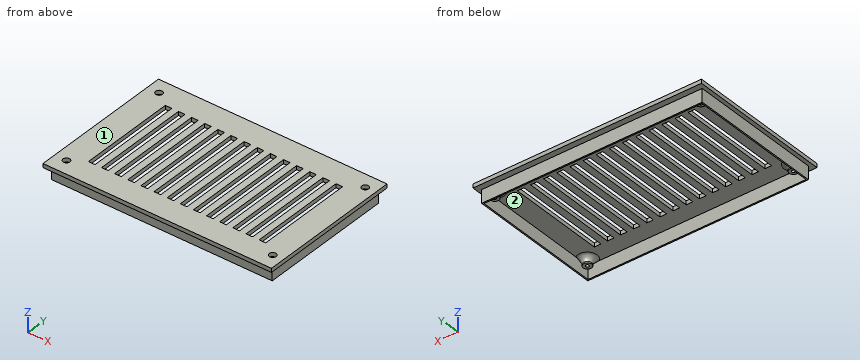
from build123d import *

# Parameters (mm, degrees)
SKETCH1_W           = 174
SKETCH1_H           = 111
SKETCH1_R           = 2.6
SKETCH1_W_2         = 5
SKETCH1_H_2         = 73.910542587
BOSS_EXTRUDE1_DEPTH = 1.5
SKETCH2_R           = 3.25
SKETCH2_R_2         = 1.25
BOSS_EXTRUDE2_DEPTH = 5
SKETCH3_W           = 168
SKETCH3_H           = 102
SKETCH3_W_2         = 166
SKETCH3_H_2         = 100
BOSS_EXTRUDE3_DEPTH = 10
FILLET1_R           = 4


with BuildPart() as part:
    # Sketch1 → Boss-Extrude1 (new, symmetric)
    with BuildSketch(Plane.XY):
        Rectangle(SKETCH1_W, SKETCH1_H)
        with Locations((-78, -44.3)):
            Circle(SKETCH1_R, mode=Mode.SUBTRACT)
        with Locations((-78, 44.7)):
            Circle(SKETCH1_R, mode=Mode.SUBTRACT)
        with Locations((79, 44.7)):
            Circle(SKETCH1_R, mode=Mode.SUBTRACT)
        with Locations((79, -44.3)):
            Circle(SKETCH1_R, mode=Mode.SUBTRACT)
        with Locations((-54.5, -0.133320073)):
            Rectangle(SKETCH1_W_2, SKETCH1_H_2, mode=Mode.SUBTRACT)
        with Locations((-64.5, -0.133320073)):
            Rectangle(SKETCH1_W_2, SKETCH1_H_2, mode=Mode.SUBTRACT)
        with Locations((-44.5, -0.133320073)):
            Rectangle(SKETCH1_W_2, SKETCH1_H_2, mode=Mode.SUBTRACT)
        with Locations((-34.5, -0.133320073)):
            Rectangle(SKETCH1_W_2, SKETCH1_H_2, mode=Mode.SUBTRACT)
        with Locations((-24.5, -0.133320073)):
            Rectangle(SKETCH1_W_2, SKETCH1_H_2, mode=Mode.SUBTRACT)
        with Locations((-14.5, -0.133320073)):
            Rectangle(SKETCH1_W_2, SKETCH1_H_2, mode=Mode.SUBTRACT)
        with Locations((-4.5, -0.133320073)):
            Rectangle(SKETCH1_W_2, SKETCH1_H_2, mode=Mode.SUBTRACT)
        with Locations((5.5, -0.133320073)):
            Rectangle(SKETCH1_W_2, SKETCH1_H_2, mode=Mode.SUBTRACT)
        with Locations((15.5, -0.133320073)):
            Rectangle(SKETCH1_W_2, SKETCH1_H_2, mode=Mode.SUBTRACT)
        with Locations((25.5, -0.133320073)):
            Rectangle(SKETCH1_W_2, SKETCH1_H_2, mode=Mode.SUBTRACT)
        with Locations((35.5, -0.133320073)):
            Rectangle(SKETCH1_W_2, SKETCH1_H_2, mode=Mode.SUBTRACT)
        with Locations((45.5, -0.133320073)):
            Rectangle(SKETCH1_W_2, SKETCH1_H_2, mode=Mode.SUBTRACT)
        with Locations((55.5, -0.133320073)):
            Rectangle(SKETCH1_W_2, SKETCH1_H_2, mode=Mode.SUBTRACT)
        with Locations((65.5, -0.133320073)):
            Rectangle(SKETCH1_W_2, SKETCH1_H_2, mode=Mode.SUBTRACT)
    extrude(amount=BOSS_EXTRUDE1_DEPTH, both=True)

    # Sketch2 → Boss-Extrude2 (add)
    # profile 1 of 4: a face of its own
    with BuildSketch(Plane(origin=(0, 0, -1.5), x_dir=(-1, 0, 0), z_dir=(0, 0, -1))):
        with Locations(Location((-79, 44.7, 0), (0, 0, 180))):
            Circle(SKETCH2_R)
        with Locations((-79, 44.7)):
            Circle(SKETCH2_R_2, mode=Mode.SUBTRACT)
    # profile 2 of 4: a face of its own
    with BuildSketch(Plane(origin=(0, 0, -1.5), x_dir=(-1, 0, 0), z_dir=(0, 0, -1))):
        with Locations(Location((-79, -44.3, 0), (0, 0, 180))):
            Circle(SKETCH2_R)
        with Locations((-79, -44.3)):
            Circle(SKETCH2_R_2, mode=Mode.SUBTRACT)
    # profile 3 of 4: a face of its own
    with BuildSketch(Plane(origin=(0, 0, -1.5), x_dir=(-1, 0, 0), z_dir=(0, 0, -1))):
        with Locations(Location((78, 44.7, 0), (0, 0, 180))):
            Circle(SKETCH2_R)
        with Locations((78, 44.7)):
            Circle(SKETCH2_R_2, mode=Mode.SUBTRACT)
    # profile 4 of 4: a face of its own
    with BuildSketch(Plane(origin=(0, 0, -1.5), x_dir=(-1, 0, 0), z_dir=(0, 0, -1))):
        with Locations(Location((78, -44.3, 0), (0, 0, 180))):
            Circle(SKETCH2_R)
        with Locations((78, -44.3)):
            Circle(SKETCH2_R_2, mode=Mode.SUBTRACT)
    extrude(amount=BOSS_EXTRUDE2_DEPTH)

    # Sketch3 → Boss-Extrude3 (add)
    with BuildSketch(Plane(origin=(0, 0, -1.5), x_dir=(-1, 0, 0), z_dir=(0, 0, -1))):
        Rectangle(SKETCH3_W, SKETCH3_H)
        Rectangle(SKETCH3_W_2, SKETCH3_H_2, mode=Mode.SUBTRACT)
    extrude(amount=BOSS_EXTRUDE3_DEPTH)

    # Fillet1
    # the kernel refuses this fillet: 4 mm, written as the material it adds along each edge
    with BuildSketch(Plane(origin=(79, 44.7, -1.5), x_dir=(1, 0, 0), z_dir=(0, 1, 0))) as fillet1_piece_1_section:
        with BuildLine():
            CenterArc((3.25 + FILLET1_R, FILLET1_R), FILLET1_R, 180, 90)
            Line((3.25, FILLET1_R), (3.25, 0))
            Line((3.25, 0), (3.25 + FILLET1_R, 0))
        make_face()
    fillet1_piece_1 = revolve(axis=Axis((79, 44.7, -1.5), (0, 0, -1)), mode=Mode.PRIVATE)
    fillet1_piece_1 = split(fillet1_piece_1, bisect_by=Plane(origin=(74.608842471, 50, -2.641157529), z_dir=(0, -1, 0)), keep=Keep.TOP, mode=Mode.PRIVATE)
    fillet1_piece_1 = split(fillet1_piece_1, bisect_by=Plane(origin=(83, 44.7, -2.641157529), z_dir=(-1, 0, 0)), keep=Keep.TOP, mode=Mode.PRIVATE)
    add(fillet1_piece_1)
    with BuildSketch(Plane(origin=(79, -44.3, -1.5), x_dir=(1, 0, 0), z_dir=(0, 1, 0))) as fillet1_piece_2_section:
        with BuildLine():
            CenterArc((3.25 + FILLET1_R, FILLET1_R), FILLET1_R, 180, 90)
            Line((3.25, FILLET1_R), (3.25, 0))
            Line((3.25, 0), (3.25 + FILLET1_R, 0))
        make_face()
    fillet1_piece_2 = revolve(axis=Axis((79, -44.3, -1.5), (0, 0, -1)), mode=Mode.PRIVATE)
    fillet1_piece_2 = split(fillet1_piece_2, bisect_by=Plane(origin=(83, -44.3, -2.641059385), z_dir=(-1, 0, 0)), keep=Keep.TOP, mode=Mode.PRIVATE)
    fillet1_piece_2 = split(fillet1_piece_2, bisect_by=Plane(origin=(74.608940615, -50, -2.641059385), z_dir=(0, 1, 0)), keep=Keep.TOP, mode=Mode.PRIVATE)
    add(fillet1_piece_2)
    with BuildSketch(Plane(origin=(-78, 44.7, -1.5), x_dir=(1, 0, 0), z_dir=(0, 1, 0))) as fillet1_piece_3_section:
        with BuildLine():
            CenterArc((3.25 + FILLET1_R, FILLET1_R), FILLET1_R, 180, 90)
            Line((3.25, FILLET1_R), (3.25, 0))
            Line((3.25, 0), (3.25 + FILLET1_R, 0))
        make_face()
    fillet1_piece_3 = revolve(axis=Axis((-78, 44.7, -1.5), (0, 0, -1)), mode=Mode.PRIVATE)
    fillet1_piece_3 = split(fillet1_piece_3, bisect_by=Plane(origin=(-82.390403008, 50, -2.640403008), z_dir=(0, -1, 0)), keep=Keep.TOP, mode=Mode.PRIVATE)
    fillet1_piece_3 = split(fillet1_piece_3, bisect_by=Plane(origin=(-83, 44.7, -2.640403008), z_dir=(1, 0, 0)), keep=Keep.TOP, mode=Mode.PRIVATE)
    add(fillet1_piece_3)
    with BuildSketch(Plane(origin=(-78, -44.3, -1.5), x_dir=(1, 0, 0), z_dir=(0, 1, 0))) as fillet1_piece_4_section:
        with BuildLine():
            CenterArc((3.25 + FILLET1_R, FILLET1_R), FILLET1_R, 180, 90)
            Line((3.25, FILLET1_R), (3.25, 0))
            Line((3.25, 0), (3.25 + FILLET1_R, 0))
        make_face()
    fillet1_piece_4 = revolve(axis=Axis((-78, -44.3, -1.5), (0, 0, -1)), mode=Mode.PRIVATE)
    fillet1_piece_4 = split(fillet1_piece_4, bisect_by=Plane(origin=(-82.390309195, -50, -2.640309195), z_dir=(0, 1, 0)), keep=Keep.TOP, mode=Mode.PRIVATE)
    fillet1_piece_4 = split(fillet1_piece_4, bisect_by=Plane(origin=(-83, -44.3, -2.640309195), z_dir=(1, 0, 0)), keep=Keep.TOP, mode=Mode.PRIVATE)
    add(fillet1_piece_4)


solid = part.part
Model file for the job. Use its own axes, mm. Face numbers are marked on the shaded views. Give positions to 0.01 mm unless a question says otherwise; leave off trailing zeros. One line per item, written item: value.
Item 1: Slice it at A-A (y = -9). Give the number of separate pieces and of enclosed holes in the cut face, then the cut area to 3 significant figures.
Response values:
separate pieces: 15
enclosed holes: 0
area: 332 mm2
Item 2: Wall check: line 1 (Y direction, x = 79, z = 0.2); line 2 (Y direction, x = 60, z = -7); line 3 (X direction, y = 44.5, z = -10.5). Give the ranges that are in metal, low to high.
Response values:
line 1: -55.5 to -46.9, -41.7 to 42.1, 47.3 to 55.5
line 2: -51 to -50, 50 to 51
line 3: -84 to -83, 83 to 84
Item 3: Pin check, flat tips, straight feed: pin 1 Ø1 at (x, z) = (45.5, -9) entering from -Y; pin 2 Ø1.6 at (x, y) = (-79, 44) entering from +Z. Stop position of each tip, or through.
Response values:
pin 1: y = -51
pin 2: z = -1.5
Item 4: Two-plate mould, pull along X, no slides. Class the marked faces 1 and 2: released by +X, released by -X, zero draft, split by the parting line, or undercut.
Response values:
face 1: zero draft
face 2: undercut
